from build123d import *

# Parameters (mm, degrees)
CYLINDER003_W     = 38
CYLINDER003_H     = 120
CYLINDER003_ANGLE = 180
CYLINDER_W        = 40
CYLINDER_H        = 120
CYLINDER_ANGLE    = 180
CYLINDER002_W     = 38
CYLINDER002_H     = 10
CYLINDER002_ANGLE = 180
CYLINDER001_W     = 40
CYLINDER001_H     = 10
CYLINDER001_ANGLE = 180
CYLINDER004_W     = 40
CYLINDER004_H     = 120
CYLINDER004_ANGLE = 180
SPHERE001_ANGLE   = 180
SPHERE_ANGLE      = 180
CYLINDER006_R     = 5
CYLINDER006_DEPTH = 17
CYLINDER005_W     = 38
CYLINDER005_H     = 2.5
CYLINDER005_ANGLE = 180
BOX_W             = 76
BOX_H             = 2.5
BOX_DEPTH         = 10
BOX002_W          = 76
BOX002_H          = 120
BOX002_DEPTH      = 10
BOX001_W          = 80
BOX001_H          = 120
BOX001_DEPTH      = 10


with BuildPart() as obj1:
    # Cylinder003 → Cylinder003 (revolve)
    with BuildSketch(Plane(origin=(40, 20, 40), x_dir=(1, 0, 0), z_dir=(0, 0, -1))):
        with Locations((19, 60)):
            Rectangle(CYLINDER003_W, CYLINDER003_H)
    revolve(axis=Axis((40, 20, 40), (0, -1, 0)), revolution_arc=CYLINDER003_ANGLE)


with BuildPart() as obj2:
    # Cylinder → Cylinder (revolve)
    with BuildSketch(Plane(origin=(40, 20, 40), x_dir=(1, 0, 0), z_dir=(0, 0, -1))):
        with Locations((20, 60)):
            Rectangle(CYLINDER_W, CYLINDER_H)
    revolve(axis=Axis((40, 20, 40), (0, -1, 0)), revolution_arc=CYLINDER_ANGLE)

    # Cut001: cut obj1
    add(obj1.part, mode=Mode.SUBTRACT)


with BuildPart() as obj3:
    # Cylinder002 → Cylinder002 (revolve)
    with BuildSketch(Plane(origin=(40, -100, 30), x_dir=(-1, 0, 0), z_dir=(0, 1, 0))):
        with Locations((19, 5)):
            Rectangle(CYLINDER002_W, CYLINDER002_H)
    revolve(axis=Axis((40, -100, 30), (0, 0, 1)), revolution_arc=CYLINDER002_ANGLE)


with BuildPart() as obj4:
    # Cylinder001 → Cylinder001 (revolve)
    with BuildSketch(Plane(origin=(40, -100, 30), x_dir=(-1, 0, 0), z_dir=(0, 1, 0))):
        with Locations((20, 5)):
            Rectangle(CYLINDER001_W, CYLINDER001_H)
    revolve(axis=Axis((40, -100, 30), (0, 0, 1)), revolution_arc=CYLINDER001_ANGLE)

    # Cut003: cut obj3
    add(obj3.part, mode=Mode.SUBTRACT)


with BuildPart() as cylinder004:
    # Cylinder004 → Cylinder004 (revolve)
    with BuildSketch(Plane(origin=(40, 20, 40), x_dir=(1, 0, 0), z_dir=(0, 0, -1))):
        with Locations((20, 60)):
            Rectangle(CYLINDER004_W, CYLINDER004_H)
    revolve(axis=Axis((40, 20, 40), (0, -1, 0)), revolution_arc=CYLINDER004_ANGLE)


with BuildPart() as obj5:
    # Sphere001 → Sphere001 (revolve)
    with BuildSketch(Plane(origin=(40, -100, 40), x_dir=(1, 0, 0), z_dir=(0, 0, -1))):
        with BuildLine():
            ThreePointArc((0, -38), (38, 0), (0, 38))
            Line((0, 38), (0, -38))
        make_face()
    revolve(axis=Axis((40, -100, 40), (0, -1, 0)), revolution_arc=SPHERE001_ANGLE)


with BuildPart() as obj6:
    # Sphere → Sphere (revolve)
    with BuildSketch(Plane(origin=(40, -100, 40), x_dir=(1, 0, 0), z_dir=(0, 0, -1))):
        with BuildLine():
            ThreePointArc((0, -40), (40, 0), (0, 40))
            Line((0, 40), (0, -40))
        make_face()
    revolve(axis=Axis((40, -100, 40), (0, -1, 0)), revolution_arc=SPHERE_ANGLE)

    # Cut002: cut obj5
    add(obj5.part, mode=Mode.SUBTRACT)

    # Cut004: cut Cylinder004
    add(cylinder004.part, mode=Mode.SUBTRACT)


with BuildPart() as agujero:
    # Cylinder006 → Cylinder006 (new body)
    with BuildSketch(Plane(origin=(40, 24, 40), x_dir=(1, 0, 0), z_dir=(0, -1, 0))):
        Circle(CYLINDER006_R)
    extrude(amount=CYLINDER006_DEPTH)


with BuildPart() as soporte_para_superior:
    # Cylinder005 → Cylinder005 (revolve)
    with BuildSketch(Plane(origin=(40, 17.5, 40), x_dir=(-1, 0, 0), z_dir=(0, 0, -1))):
        with Locations((19, 1.25)):
            Rectangle(CYLINDER005_W, CYLINDER005_H)
    revolve(axis=Axis((40, 17.5, 40), (0, 1, 0)), revolution_arc=CYLINDER005_ANGLE)


with BuildPart() as soporte_con_agujero:
    # Box → Box (new body)
    with BuildSketch(Plane(origin=(2, 17.5, 30), x_dir=(1, 0, 0), z_dir=(0, 0, 1))):
        with Locations((38, 1.25)):
            Rectangle(BOX_W, BOX_H)
    extrude(amount=BOX_DEPTH)

    # Fusion: union Soporte para superior
    add(soporte_para_superior.part)

    # Cut005: cut Agujero
    add(agujero.part, mode=Mode.SUBTRACT)


with BuildPart() as obj7:
    # Box002 → Box002 (new body)
    with BuildSketch(Plane(origin=(2, -100, 30), x_dir=(1, 0, 0), z_dir=(0, 0, 1))):
        with Locations((38, 60)):
            Rectangle(BOX002_W, BOX002_H)
    extrude(amount=BOX002_DEPTH)


with BuildPart() as obj8:
    # Box001 → Box001 (new body)
    with BuildSketch(Plane(origin=(0, -100, 30), x_dir=(1, 0, 0), z_dir=(0, 0, 1))):
        with Locations((40, 60)):
            Rectangle(BOX001_W, BOX001_H)
    extrude(amount=BOX001_DEPTH)

    # Cut: cut obj7
    add(obj7.part, mode=Mode.SUBTRACT)

    # Fusion001: union obj2, obj4, obj6, Soporte con agujero
    add(obj2.part)
    add(obj4.part)
    add(obj6.part)
    add(soporte_con_agujero.part)


solid = obj8.part
Design review of the part built by this model. Coordinates are the model's own, in mm. A direction names the side the tool comes from. Give positions to 0.01 mm unless a question says otherwise; leave off trailing zeros. Write each loop counter-clockwise with the first axis right and the second up, starting at its lowest first coordinate (ties: lowest second). Pieces come first, ordered by that corner, then holes. Notation, with made-up numbers: M -12.5,-1 L 35.5,-1 A17 cw 35.5,23 Z; hole C 41,-18.75 d5. An arc over 180 degrees is marked long. Answer as a JSON object with one key per item and string values. Group by question number.
1) We need section D-D (x = 9). Give the boundary of the cut face in (y, z).
2) For line 1 along X through (y, z) = (18, 40); line 2 along Z through (x, y) = (40, 19.15); line 3 along Z through (x, y) = (39, -40), list the stretches that pass through material, from the lowest coordinate up.
3) We need section C-C (y = -60). Give the boundary of the cut face in (x, z), and give its area (3 significant figures).
4) We need section A-A (x = 40). Give the boundary of the cut face in (y, z), and give its area (3 significant figures).
5) Clearance check with flat-ended pins moving along their axes: pin 1 Ø5 at (x, z) = (66.5, 49) entering from -Y; pin 2 Ø8 at (y, z) = (-30, 36) entering from -X; pin 3 Ø10 at (x, z) = (20, 44.5) entering from -Y; pin 4 Ø3 at (y, z) = (-36, 61.5) entering from +X. State where each tip first meets the part, or that it passes through.
6) We need section B-B (z = 48). Give the boundary of the cut face in (x, y).
7) Tool access review of faces 1 (the face through (78, -42, 35)), 2 (the face through (39.12, -139.99, 35.07)): name each direction out of +Z, -Z, +X, -X, +Y, -Y from which nothing blocks a thin tool from reaching the whole face with its end or side.
8) Mouldability with a two-part tool opening along Z and no side actions: class faces 3 (the face through (40.84, -42.07, 77.99)), 4 (the face through (0, -41, 35)), 5 (the face through (36, 19, 43)), 6 (the face through (40.88, -40.84, 79.99)) as released by +Z, released by -Z, zero draft, split by the parting line, or undercut.
Answer key:
{
 "1": {"outline": "M -125.28,30 L -121.98,30 L -121.98,40 A21.98 cw -100,61.98 L 17.5,61.98 L 17.5,30 L 20,30 L 20,65.28 L -100,65.28 A25.28 ccw -125.28,40 Z"},
 "2": {"line 1": "x = 0 to 35, 45 to 80", "line 2": "z = 30 to 35, 45 to 80", "line 3": "z = 77.99 to 79.99"},
 "3": {"outline": "M 0,30 L 2,30 L 2,40 A38 cw 78,40 L 78,30 L 80,30 L 80,40 A40 ccw 0,40 Z", "area": "285 mm²"},
 "4": {"outline": "M -140,30 L -138,30 L -138,40 A38 cw -100,78 L 17.5,78 L 17.5,45 L 20,45 L 20,80 L -100,80 A40 ccw -140,40 Z; M 17.5,30 L 20,30 L 20,35 L 17.5,35 Z", "area": "478 mm²"},
 "5": {"pin 1": "stops at y = -130.83", "pin 2": "stops at x = 0", "pin 3": "stops at y = -136.87", "pin 4": "stops at x = 74.64"},
 "6": {"outline": "M 0.81,-100 A39.19 ccw 79.19,-100 L 79.19,20 L 0.81,20 Z; hole M 2.85,-100 A37.15 ccw 77.15,-100 L 77.15,17.5 L 2.85,17.5 Z"},
 "7": {"face 1": "-Z", "face 2": "+Z, -Z, -Y"},
 "8": {"face 3": "released by -Z", "face 4": "zero draft", "face 5": "undercut", "face 6": "released by +Z"}
}
